Could you check a few things on this model? Use its own coordinates, in mm. A direction names the side the tool comes from. Coordinates: 2 decimals unless noted, no trailing zeros. Order: outer loops, then holes, each group sorted by start corner. A loop starts at its lowest first (then second) coordinate and runs counter-clockwise, first axis right, second up. Notation, with made-up numbers: (74, -30) - (81, -30) arc R28 ccw to (81, -8) - close; hole circle Ø2 at (10, 82). An arc over 180 degrees is marked (long way). Answer as a JSON object with one key per item and string values. Group by question number.
(1) Imagine slicing it at D-D, the plane x = -48. Write out the boundary of the cut face in (y, z).
(2) We'd pull the mould along Z, two halves only. Please class faces 1 (the cylindrical face through (-16.31, -23.83, 46.87)), 2 (the flat face through (-35, -23, 51.3)), 3 (the flat face through (-14, 0, 27)): pulls with the +Z half, pulls with the -Z half, needs draft (parallel to the pull), parting line crosses it, or undercut.
(3) Imagine slicing it at C-C, the plane z = 24.5. Write out the boundary of the cut face in (x, y).
(4) Imagine slicing it at B-B, the plane y = -6. Write out the boundary of the cut face in (x, z), and give its area (3 significant figures).
(5) Which directions (+Z, -Z, +X, -X, +Y, -Y) give clear straight access to the entire face, cutting with the end or side of a thin tool? Please do faces 4 (the flat face through (-44.811, -23, 2)), 5 (the flat face through (-11.811, -23, 28)), 6 (the flat face through (-40, -23, 48.3)).
(6) Please list where these lines run through material, in increasing order: probe 1 along Z at (x, y) = (-36, -13.5); probe 2 along X at (y, z) = (-29, 23); probe 3 along Z at (x, y) = (-57, -9).
(7) Imagine slicing it at A-A, the plane x = -35. Write out the boundary of the cut face in (y, z).
(8) Will these pins go through, and if not, where does the flat tip stop? P1, Ø6, axis at x = -35.5, z = 45, coming from the -Y side; P2, Ø1, axis at y = -41.5, z = 25.5, coming from the -X side; P3, Ø1.5, axis at y = -34.5, z = 1, coming from the -X side.
from build123d import *

# Parameters (mm, degrees)
F1_DEPTH  = 47
F2_R      = 5
F3_R      = 5
F1_FACE_W = 47
F1_FACE_H = 3
F4_DEPTH  = 15


with BuildPart() as f1:
    # F0 (on Front) → F1 (new body)
    with BuildSketch(Plane.XZ):
        Polygon((-11.811316, 51.3), (-44.811316, 51.3), (-44.811316, 48.3), (-14.811316, 48.3), (-14.811316, 3), (-44.811316, 3), (-44.811316, 0), (-11.811316, 0), align=None)
    extrude(amount=F1_DEPTH)

    # F2
    f2_edges = [f1.edges().sort_by_distance(p)[0] for p in [
        (-14.811316, -23.5, 3),
        (-14.811316, -23.5, 48.3),
    ]]
    fillet(f2_edges, radius=F2_R)

    # F3
    f3_edges = [f1.edges().sort_by_distance(p)[0] for p in [
        (-11.811316, -23.5, 0),
    ]]
    fillet(f3_edges, radius=F3_R)

    # F1_face (on face) → F4 (join)
    with BuildSketch(Plane(origin=(-44.811316, -23.5, 49.8), x_dir=(0, -1, 0), z_dir=(-1, 0, 0))):
        Rectangle(F1_FACE_W, F1_FACE_H)
    extrude(amount=F4_DEPTH)


solid = f1.part
Result set:
{
 "1": {"outline": "(-47, 48.3) - (0, 48.3) - (0, 51.3) - (-47, 51.3) - close"},
 "2": {"face 1": "undercut", "face 2": "pulls with the +Z half", "face 3": "needs draft"},
 "3": {"outline": "(-14.81, -47) - (-11.81, -47) - (-11.81, 0) - (-14.81, 0) - close"},
 "4": {"outline": "(-59.81, 48.3) - (-19.81, 48.3) arc R5 cw to (-14.81, 43.3) - (-14.81, 8) arc R5 cw to (-19.81, 3) - (-44.81, 3) - (-44.81, 0) - (-16.81, 0) arc R5 ccw to (-11.81, 5) - (-11.81, 51.3) - (-59.81, 51.3) - close", "area": "384 mm^2"},
 "5": {"face 4": "-Z, -X, +Y, -Y", "face 5": "+Z, -Z, +X, +Y, -Y", "face 6": "-X, +Y, -Y"},
 "6": {"probe 1": "z = 0 to 3, 48.3 to 51.3", "probe 2": "x = -14.81 to -11.81", "probe 3": "z = 48.3 to 51.3"},
 "7": {"outline": "(-47, 0) - (0, 0) - (0, 3) - (-47, 3) - close; (-47, 48.3) - (0, 48.3) - (0, 51.3) - (-47, 51.3) - close"},
 "8": {"P1": "passes through", "P2": "stops at x = -14.81", "P3": "stops at x = -44.81"}
}
